```python
from build123d import *

# Parameters (mm, degrees)
BOSS_EXTRUDE1_DEPTH = 12
SKETCH3_R           = 2.4
CUT_EXTRUDE1_DEPTH  = 8.5
FILLET1_R           = 6


with BuildPart() as part:
    # Sketch1 → Boss-Extrude1 (new body)
    with BuildSketch(Plane(origin=(0, 0, 0), x_dir=(1, 0, 0), z_dir=(0, 1, 0))):
        Polygon((-50, 17.7), (50, 17.7), (50, 13.7), (27.895, 0), (-27.895, 0), (-50, 13.7), align=None)
    extrude(amount=BOSS_EXTRUDE1_DEPTH)

    # Sketch3 → Cut-Extrude1 (cut)
    with BuildSketch(Plane.XY):
        with Locations((-23.91, 8)):
            Circle(SKETCH3_R)
        with Locations(Location((23.91, 8, 0), (0, 0, 180))):
            Circle(SKETCH3_R)
    extrude(amount=-CUT_EXTRUDE1_DEPTH, mode=Mode.SUBTRACT)

    # Fillet1
    # the kernel refuses this fillet: 6 mm, written as the material it takes off along each edge
    with BuildSketch(Plane(origin=(50, -14.142135624, -17.7), x_dir=(-1, 0, 0), z_dir=(0, 1, 0))) as fillet1_piece_1:
        with BuildLine():
            CenterArc((5.656854249, 6), FILLET1_R, 199.471220634, 70.528779366)
            Line((0, 4), (-0.113137085, 3.96))
            ThreePointArc((-0.113137085, 3.96), (-0.12, 2), (-0.12, 0))
            Line((-0.12, 0), (0, -0.12))
            Line((0, -0.12), (5.656854249, -0.12))
            Line((5.656854249, -0.12), (5.656854249, 0))
        make_face()
    extrude(amount=40.284271247, mode=Mode.SUBTRACT)
    with BuildSketch(Plane(origin=(-50, -14.142135624, -17.7), x_dir=(1, 0, 0), z_dir=(0, 1, 0))) as fillet1_piece_2:
        with BuildLine():
            CenterArc((5.656854249, -6), FILLET1_R, 90, 70.528779366)
            Line((0, -4), (-0.113137085, -3.96))
            ThreePointArc((-0.113137085, -3.96), (-0.12, -2), (-0.12, 0))
            Line((-0.12, 0), (0, 0.12))
            Line((0, 0.12), (5.656854249, 0.12))
            Line((5.656854249, 0.12), (5.656854249, 0))
        make_face()
    extrude(amount=40.284271247, mode=Mode.SUBTRACT)


solid = part.part
```
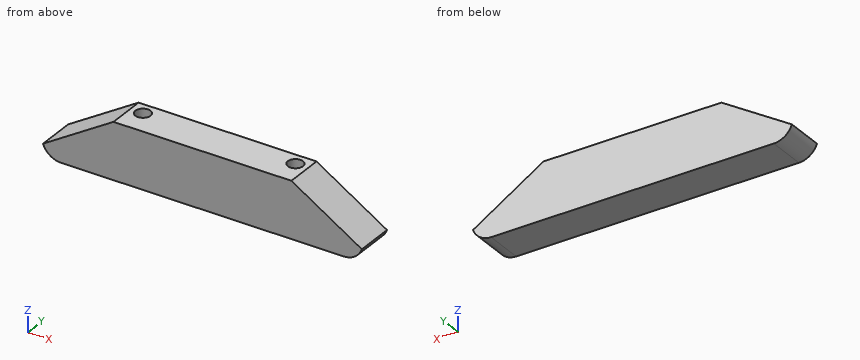
For this review, take the finished solid that the model builds, in its own axes (mm). Coordinates: 2 decimals unless noted, no trailing zeros. Loops run counter-clockwise (first coordinate to the right, second up) from the corner with the lowest first, then second, coordinate; pieces in that order, holes last.
1. Add section B-B, the plane y = 8. Give the boundary of the cut face in (x, z) (3 decimals), then the cut area to 3 significant figures.
2. For line 1 (Y direction, x = 23.91, z = -5); line 2 (X direction, y = 7, z = -3.25); line 3 (X direction, y = 7.5, z = -7.25), list the stretches that pass through material, from the lowest coordinate up.
3. Add section D-D, the plane y = 1. Give the boundary of the cut face in (x, z) (3 decimals), then the cut area to 3 significant figures.
4. Add section C-C, the plane z = -5.5. Give the boundary of the cut face in (x, y), then the cut area to 3 significant figures.
5. Add section A-A, the plane x = 23.91. Give the boundary of the cut face in (y, z), then the cut area to 3 significant figures.
Result:
1. outline: (-50, -13.7) arc R6 ccw to (-44.343, -17.7) - (44.343, -17.7) arc R6 ccw to (50, -13.7) - (27.895, 0) - (26.31, 0) - (26.31, -8.5) - (21.51, -8.5) - (21.51, 0) - (-21.51, 0) - (-21.51, -8.5) - (-26.31, -8.5) - (-26.31, 0) - (-27.895, 0) - close
1. area: 1,370 mm2
2. line 1: y = 0 to 5.6, 10.4 to 12
2. line 2: x = -33.14 to -26.09, -21.73 to 21.73, 26.09 to 33.14
2. line 3: x = -39.59 to -26.26, -21.56 to 21.56, 26.26 to 39.59
3. outline: (-50, -13.7) arc R6 ccw to (-44.343, -17.7) - (44.343, -17.7) arc R6 ccw to (50, -13.7) - (27.895, 0) - (-27.895, 0) - close
3. area: 1,450 mm2
4. outline: (-36.77, 0) - (36.77, 0) - (36.77, 12) - (-36.77, 12) - close; hole circle Ø4.8 at (-23.91, 8); hole circle Ø4.8 at (23.91, 8)
4. area: 846 mm2
5. outline: (0, -17.7) - (12, -17.7) - (12, 0) - (10.4, 0) - (10.4, -8.5) - (5.6, -8.5) - (5.6, 0) - (0, 0) - close
5. area: 172 mm2
